Here's how the part is built. I have some questions about the finished solid (model axes, mm). A direction names the side the tool comes from. Coordinates: 2 decimals unless noted, no trailing zeros. Loops run counter-clockwise (first coordinate to the right, second up) from the corner with the lowest first, then second, coordinate; pieces in that order, holes last. Notation, with made-up numbers: M -30,78 L 10,78 A15 cw 10,105 Z; hole C 31,78.25 d3. An arc over 180 degrees is marked long. Use one line per item in the form item = value. Start each with the question number.
(1) Imagine slicing it at A-A, the plane z = 25. Please give me the cut outline in (x, y).
(2) Imagine slicing it at D-D, the plane z = 38.5. Please give me the cut outline in (x, y).
(3) Will these pins go through, and if not, where does the flat tip stop? P1, Ø1.5, axis at y = 33, z = 38, coming from the -X side; P2, Ø6, axis at x = -0.5, z = 9.5, coming from the +Y side; P3, Ø6, axis at y = 25, z = 10, coming from the +X side; P4, Ø12, axis at x = -41.5, z = 30, coming from the +Y side.
(4) Please list where these lines run through material, in increasing order: L1, parallel to Z at x = 32, y = 4; L2, parallel to Z at x = -35, y = 25.5; L3, parallel to Y at x = -13.5, z = 7.
(5) On a 3-axis mill with a long thin cutter (end or side, diameter ignored), from which of +Z, -Z, +X, -X, +Y, -Y can I reach the whole of each face in a straight line? I mean faces 4 (the flat face through (25, 7, 15)), 5 (the flat face through (3, 7, 0)). Say none if no direction works.
(6) Thinking about a two-plate mould opening in Z: for faces 1 (the cylindrical face through (-59.976, 24.164, 26.099)), 2 (the cylindrical face through (0.163, 7.395, 25.22)), 3 (the flat face through (-24, 40, 14)), which applies, +Z half, -Z half, draft (parallel to the pull), parting line (faces both ways), or undercut?
(7) Imagine slicing it at C-C, the plane x = -43. Please give me the cut outline in (y, z).
Autodesk Inventor part; units mm, degrees
ref_plane "YZ Plane" through (0, 0, 0) normal (1, 0, 0) x (0, 1, 0)
ref_plane "XZ Plane" through (0, 0, 0) normal (0, 1, 0) x (-1, 0, 0)
ref_plane "XY Plane" through (0, 0, 0) normal (0, 0, 1) x (1, 0, 0)
sketch "Sketch4" plane through (0, 0, 0) normal (0, 1, 0) x (-1, 0, 0)
  line L0 (-40.1608, 0) -> (34.8392, 0)
  line L1 (34.8392, 0) -> (34.8392, 50)
  line L2 (34.8392, 50) -> (-40.1608, 50)
  line L3 (-40.1608, 50) -> (-40.1608, 0)
  point P0 (0, 0)
  point P1 (0, 0)
  dimension "d3" = 75
  dimension "d4" = 50
extrude "Extrusion1" add sketch "Sketch4" along normal blind 15
sketch "Sketch5" plane through (0, 0, 0) normal (0, -1, 0) x (1, 0, 0)
  point P0 (0, 0)
sketch "Sketch7" plane through (0, 0, 0) normal (0, -1, 0) x (1, 0, 0)
  line L0 (-34.8392, 0) -> (-34.8392, 50)
  circle A0 centre (-35, 25) radius 25.0005
  point P0 (0, 0)
extrude "Extrusion3" add sketch "Sketch7" against normal blind 40
sketch "Sketch8" plane through (-35, 40, 25) normal (0, 1, 0) x (1, 0, 0)
  circle A0 centre (0, 0) radius 15
  point P0 (35, 25)
  dimension "d11" = 30
extrude "Extrusion4" cut sketch "Sketch8" against normal through all
sketch "Sketch9" plane through (0, 15, 0) normal (0, 1, 0) x (1, 0, 0)
  line L0 (40.1608, -50) -> (40.1608, 0)
  line L1 (40.1608, 0) -> (-34.8392, 0)
  point P0 (0, 0)
  point P1 (10.1608, -25)
  dimension "d14" = 30
  dimension "d15" = 25
hole "Hole1" at (10.1608, 15, 25) direction (0, -1, 0) diameter 20 end through all
sketch "Sketch10" plane through (40.1608, 0, 50) normal (1, 0, 0) x (0, 0, -1)
  line L0 (15, 0) -> (15, 15)
  line L1 (15, 0) -> (35, 0)
  line L2 (35, 0) -> (35, 15)
  line L3 (35, 15) -> (15, 15)
  line L4 (15, 15) -> (15, 0)
  point P0 (50, 0)
extrude "Extrusion5" cut sketch "Sketch10" against normal up to surface
properties part number "Assignment 3 - Locator"
Answer:
q1.outline = M -60,0 L -50,0 L -50,40 L -60,40 Z; M -20,0 L 0.16,0 L 0.16,15 L -10,15 L -10,40 L -20,40 Z
q2.outline = M -56.04,0 L -41.54,0 L -41.54,40 L -56.04,40 Z; M -28.46,0 L 40.16,0 L 40.16,15 L -13.96,15 L -13.96,40 L -28.46,40 Z
q3.P1 = -56.79
q3.P2 = 15
q3.P3 = -13.07
q3.P4 = through
q4.L1 = 0 to 15, 35 to 50
q4.L2 = 0 to 10, 40 to 50
q4.L3 = 0 to 15
q5.face_4 = +X, +Y, -Y
q5.face_5 = -Z, +X, -X, +Y, -Y
q6.face_1 = parting line
q6.face_2 = undercut
q6.face_3 = draft
q7.outline = M 0,1.31 L 40,1.31 L 40,12.31 L 0,12.31 Z; M 0,37.69 L 40,37.69 L 40,48.69 L 0,48.69 Z
